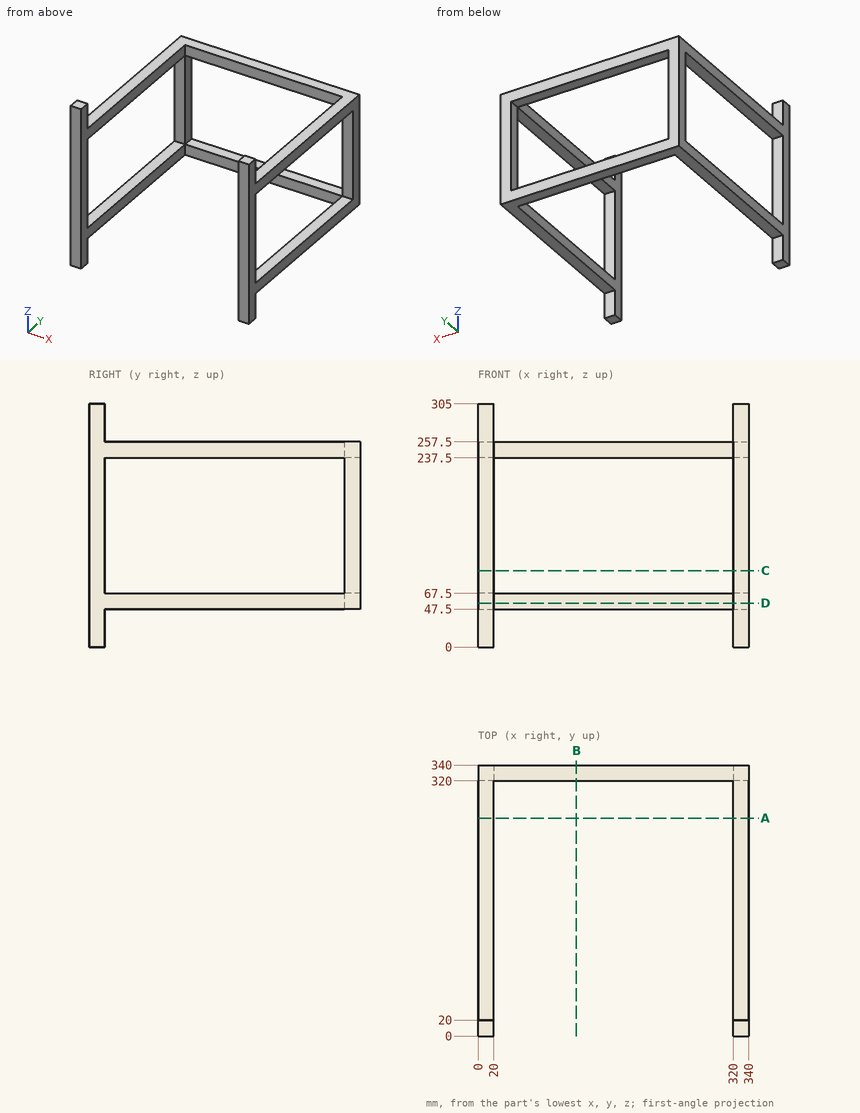
Here's the drawing with two shaded views (mm, measured from the low corner). I have some questions. Coordinates: 2 decimals unless noted, no trailing zeros. Order: outer loops, then holes, each group sorted by start corner. A loop starts at its lowest first (then second) coordinate and runs counter-clockwise, first axis right, second up.
Item 1: If we section it at A-A, the plane y = 273.5: List the corners of the cut face in (x, z) for me, then the cut area to 3 significant figures.
Response values:
outline: (0, 47.5) - (20, 47.5) - (20, 67.5) - (0, 67.5) - close; (0, 237.5) - (20, 237.5) - (20, 257.5) - (0, 257.5) - close; (320, 47.5) - (340, 47.5) - (340, 67.5) - (320, 67.5) - close; (320, 237.5) - (340, 237.5) - (340, 257.5) - (320, 257.5) - close
area: 1,600 mm2
Item 2: I'm going to push flat-ended pins straight in: pin 1 Ø16 at (x, z) = (151.5, 247.5) entering from -Y; pin 2 Ø10 at (x, y) = (148.5, 329.5) entering from +Z; pin 3 Ø16 at (x, z) = (7.5, 280) entering from +Y. Where does each tip first touch, or does it pass through?
Response values:
pin 1: stops at y = 320
pin 2: stops at z = 257.5
pin 3: stops at y = 20
Item 3: If we section it at B-B, the plane x = 123.5: List the corners of the cut face in (y, z) for me.
Response values:
outline: (320, 47.5) - (340, 47.5) - (340, 67.5) - (320, 67.5) - close; (320, 237.5) - (340, 237.5) - (340, 257.5) - (320, 257.5) - close
Item 4: If we section it at C-C, the plane z = 96: List the corners of the cut face in (x, y) for me, then the cut area to 3 significant figures.
Response values:
outline: (0, 0) - (20, 0) - (20, 20) - (0, 20) - close; (0, 320) - (20, 320) - (20, 340) - (0, 340) - close; (320, 0) - (340, 0) - (340, 20) - (320, 20) - close; (320, 320) - (340, 320) - (340, 340) - (320, 340) - close
area: 1,600 mm2
Item 5: If we section it at D-D, the plane z = 55: List the corners of the cut face in (x, y) for me, then the cut area to 3 significant figures.
Response values:
outline: (0, 0) - (20, 0) - (20, 320) - (320, 320) - (320, 0) - (340, 0) - (340, 340) - (0, 340) - close
area: 19,600 mm2
Item 6: I need wall thicknesses on probe 1 along X at (y, z) = (284.5, 247.5). Which ranges of the line are inside material? Lowest first, please.
Response values:
probe 1: x = 0 to 20, 320 to 340
